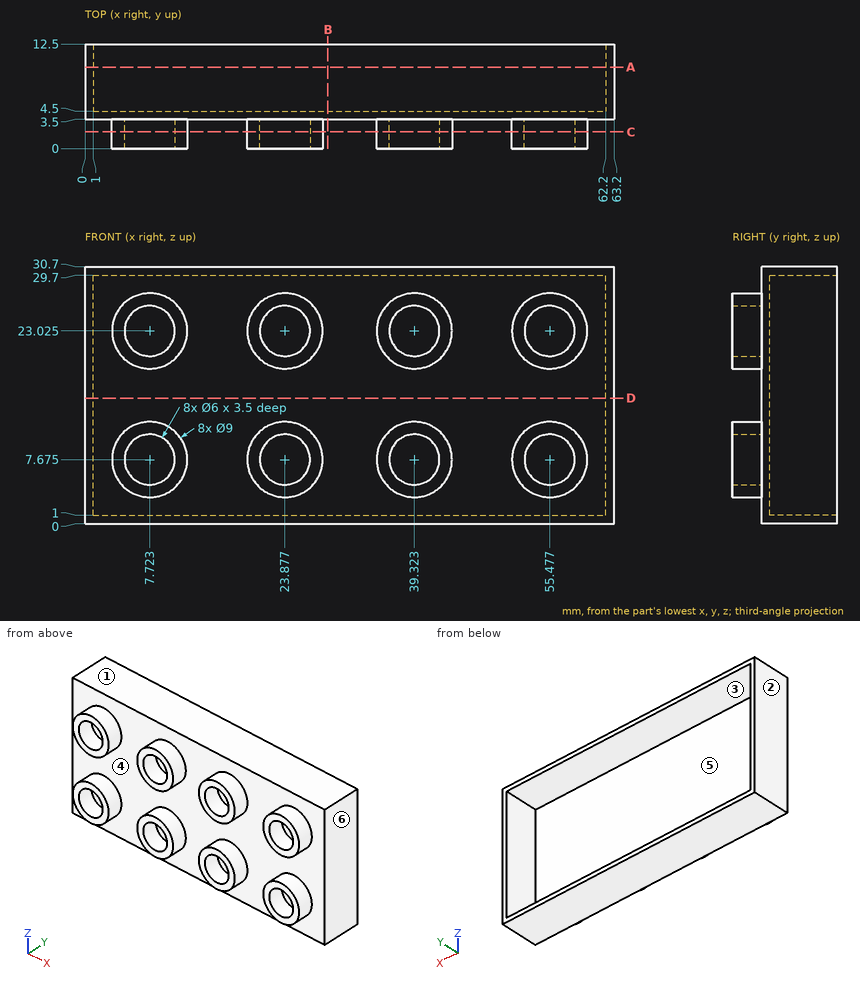
Geometry: see drawing. Coordinates: mm, zero at the bounding-box minimum. A direction names the side the tool comes from. Coordinates: 2 decimals unless noted, no trailing zeros. Order: outer loops, then holes, each group sorted by start corner. A loop starts at its lowest first (then second) coordinate and runs counter-clockwise, first axis right, second up. Notation, with made-up numbers: M 19.5,-24 L 61.5,-24 A27 ccw 61.5,5 Z; hole C 40.25,-18 d1. An arc over 180 degrees is marked long. Write item = value, one per line. Start each with the question number.
(1) Section B-B on x = 29. Output: boundary loops of the cut face in (y, z).
(2) Pull-direction query (Z, two-part tool) for the marked faces 1, 2 and 3; classes: released by +Z, released by -Z, zero draft, split by the parting line, or undercut.
(3) Section D-D on z = 15. Output: boundary loops of the cut face in (x, y).
(4) Line query: line 1 along Z through (x, y) = (27, 7.5); line 2 along X through (y, z) = (8.5, 10.5); line 3 along X through (y, z) = (2.5, 4.5) (1 decimal). Output: solid intervals per line, ascending. Write a range as [from, to].
(5) Section A-A on y = 9.75. Output: boundary loops of the cut face in (x, z).
(6) Section C-C on y = 2. Give the number of separate pieces and of enclosed holes in the cut face.
(7) First-contact query: P1, Ø10, axis at x = 39.5, z = 4.5, coming from the +Y side; P2, Ø1.8, axis at x = 55.5, z = 7.5, coming from the -Y side; P3, Ø5, axis at x = 7.72, z = 23.02, coming from the +Y side; P4, Ø2, axis at x = 51.5, y = 1.5, coming from the +Z side. Flat tips, straight axial feed; report the tip coordinate or a pass-through.
(8) Reachability of the marked faces 4, 5 and 6 from +Z, -Z, +X, -X, +Y, -Y: full face, straight path, thin tool, end or side. Return the list, or none.
Result set:
q1.outline = M 3.5,0 L 12.5,0 L 12.5,1 L 4.5,1 L 4.5,29.7 L 12.5,29.7 L 12.5,30.7 L 3.5,30.7 Z
q2.face_1 = released by +Z
q2.face_2 = zero draft
q2.face_3 = undercut
q3.outline = M 0,3.5 L 63.2,3.5 L 63.2,12.5 L 62.2,12.5 L 62.2,4.5 L 1,4.5 L 1,12.5 L 0,12.5 Z
q4.line_1 = [0, 1], [29.7, 30.7]
q4.line_2 = [0, 1], [62.2, 63.2]
q4.line_3 = [4.5, 10.9], [20.7, 27.1], [36.1, 42.5], [52.3, 58.7]
q5.outline = M 0,0 L 63.2,0 L 63.2,30.7 L 0,30.7 Z; hole M 1,1 L 62.2,1 L 62.2,29.7 L 1,29.7 Z
q6.separate_pieces = 8
q6.enclosed_holes = 8
q7.P1 = 12.5
q7.P2 = 3.5
q7.P3 = 4.5
q7.P4 = 26.4
q8.face_4 = -Y
q8.face_5 = +Y
q8.face_6 = +Z, -Z, +X, +Y, -Y
